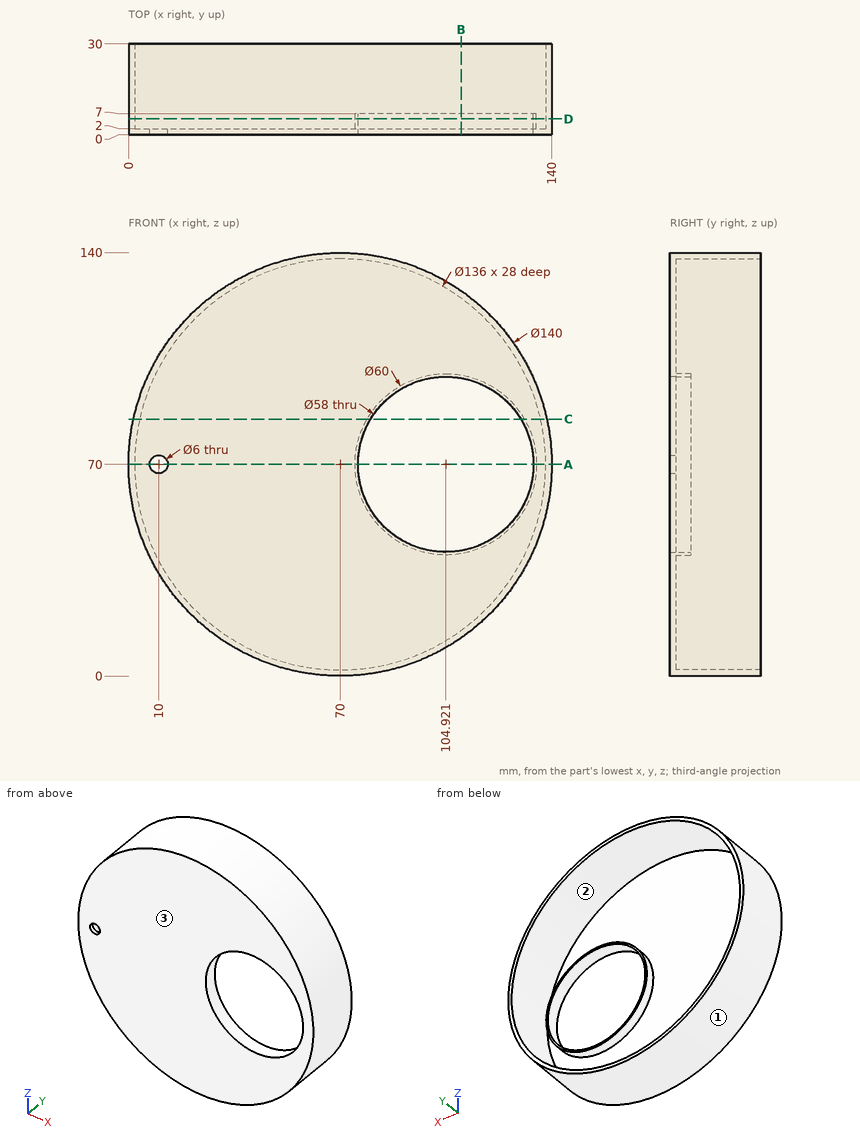
Could you check a few things on this drawing? It's one solid part, dimensions in mm from its lowest x, y, z. Round coordinates to 2 decimals unless told otherwise and drop trailing zeros. Loops run counter-clockwise (first coordinate to the right, second up) from the corner with the lowest first, then second, coordinate; pieces in that order, holes last. Notation, with made-up numbers: M 87,69.5 L 117,69.5 A20 cw 117,107.5 Z; hole C 83.5,84 d2. An arc over 180 degrees is marked long. Write each question's results on one line, items separated by ' | '. Start each with the question number.
(1) I want a section at C-C (z = 85). Please give me the cut outline in (x, y) (1 decimal).
(2) I want a section at A-A (z = 70). Please give me the cut outline in (x, y).
(3) I want a section at B-B (x = 110). Please give me the cut outline in (y, z) (1 decimal), then the cut area to 3 significant figures.
(4) I want a section at D-D (y = 5.25). Please give me the cut outline in (x, z), then the cut area to 3 significant figures.
(5) Will these pins go through, and if not, where does the flat tip stop? P1, Ø12, axis at y = 25, z = 111, coming from the +X side; P2, Ø5, axis at x = 41.5, z = 112, coming from the +Y side; P3, Ø1, axis at x = 21.5, y = 7, coming from the -Z side; P4, Ø5.5, axis at x = 10, z = 70, coming from the +Y side.
(6) If I drill on probe 1 along X at (y, z) = (4, 70); probe 2 along X at (y, z) = (1.25, 70); probe 3 along Y at (x, z) = (114.5, 114), over which ranges is the centre line in solid material (lowest first)? Write a range as from..to.
(7) Thinking about a two-plate mould opening in X: for the marked faces 1, 2 and 3, which applies, pulls with the +X half, pulls with the -X half, needs draft (parallel to the pull), parting line crosses it, or undercut?
Solved:
1) outline: M 1.6,0 L 80.1,0 L 80.1,7 L 78.9,7 L 78.9,2 L 3.7,2 L 3.7,30 L 1.6,30 Z; M 129.7,0 L 138.4,0 L 138.4,30 L 136.3,30 L 136.3,2 L 130.9,2 L 130.9,7 L 129.7,7 Z
2) outline: M 0,0 L 7,0 L 7,2 L 2,2 L 2,30 L 0,30 Z; M 13,0 L 75.92,0 L 75.92,7 L 74.92,7 L 74.92,2 L 13,2 Z; M 133.92,0 L 140,0 L 140,30 L 138,30 L 138,2 L 134.92,2 L 134.92,7 L 133.92,7 Z
3) outline: M 0,12.6 L 30,12.6 L 30,15 L 2,15 L 2,40.4 L 7,40.4 L 7,41.4 L 0,41.4 Z; M 0,98.6 L 7,98.6 L 7,99.6 L 2,99.6 L 2,125 L 30,125 L 30,127.4 L 0,127.4 Z | area: 263 mm²
4) outline: C 70,70 d140; C 104.92,70 d60; hole C 70,70 d136; hole C 104.92,70 d58 | area: 1,050 mm²
5) P1: stops at x = 130.62 | P2: stops at y = 2 | P3: stops at z = 19.05 | P4: passes through
6) probe 1: x = 0..2, 74.92..75.92, 133.92..134.92, 138..140 | probe 2: x = 0..7, 13..75.92, 133.92..140 | probe 3: y = 0..2
7) face 1: parting line crosses it | face 2: undercut | face 3: needs draft
